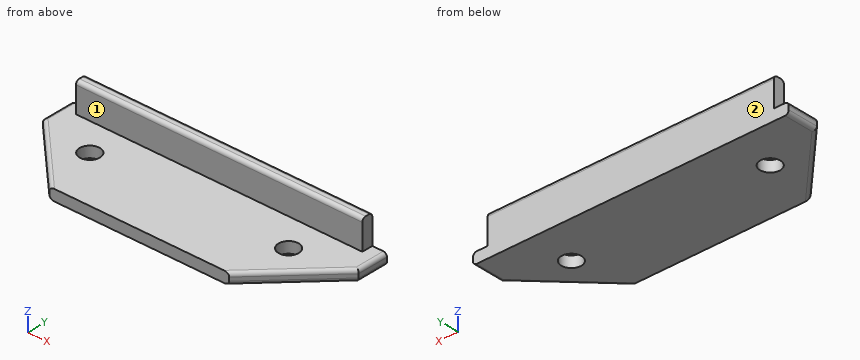
```python
from build123d import *

# Parameters (mm, degrees)
BOSS_EXTRUDE1_DEPTH       = 9.525
SKETCH2_W                 = 247.649999748
SKETCH2_H                 = 9.52499999
BOSS_EXTRUDE2_DEPTH       = 25.4
M16_CLEARANCE_HOLE1_D     = 17.462499982
M16_CLEARANCE_HOLE1_DEPTH = 34.925
FILLET1_R                 = 3.175


with BuildPart() as part:
    # Sketch1 → Boss-Extrude1 (new body)
    with BuildSketch(Plane.XY.offset(-7.9375)):
        Polygon((136.524999861, 15.874999984), (136.524999861, 42.862499956), (-136.524999861, 42.862499956), (-136.524999861, 15.874999984), (-77.787499921, -42.862499956), (77.787499921, -42.862499956), align=None)
    extrude(amount=-BOSS_EXTRUDE1_DEPTH)

    # Sketch2 → Boss-Extrude2 (add)
    with BuildSketch(Plane.XY.offset(-7.9375)):
        with Locations((0, 38.099999961)):
            Rectangle(SKETCH2_W, SKETCH2_H)
    extrude(amount=BOSS_EXTRUDE2_DEPTH)

    # M16 Clearance Hole1
    with Locations(Plane(origin=(0, 0, -17.4625), x_dir=(-1, 0, 0), z_dir=(0, 0, -1))):
        with Locations((-85.978999912, 4.762499995), (85.978999912, 4.762499995)):
            Hole(M16_CLEARANCE_HOLE1_D / 2, depth=M16_CLEARANCE_HOLE1_DEPTH)

    # Fillet1
    fillet1_edges = [part.edges().sort_by_distance(p)[0] for p in [
        (-136.524999861, 29.36874997, -17.4625),
        (-107.156249891, -13.493749986, -17.4625),
        (0, 33.337499966, 17.4625),
        (0, 42.862499956, 17.4625),
        (107.156249891, -13.493749986, -17.4625),
        (-107.156249891, -13.493749986, -7.9375),
        (-136.524999861, 29.36874997, -7.9375),
        (136.524999861, 29.36874997, -17.4625),
        (136.524999861, 29.36874997, -7.9375),
        (107.156249891, -13.493749986, -7.9375),
    ]]
    fillet(fillet1_edges, radius=FILLET1_R)


solid = part.part
```
Geometry check sheet. Reference: the model listing, model coordinates, mm. Face numbers are marked on the shaded views. A direction names the side the tool comes from. Round coordinates to 2 decimals unless told otherwise and drop trailing zeros. Order: outer loops, then holes, each group sorted by start corner. A loop starts at its lowest first (then second) coordinate and runs counter-clockwise, first axis right, second up. Notation, with made-up numbers: (54.25, 40.5) -> (107.25, 40.5) arc R19 ccw to (107.25, 66.5) -> close; hole circle Ø10 at (68, 77.25). An arc over 180 degrees is marked (long way). Return JSON: item names as keys, results as strings. Group by question number.
Q1. Material ranges on probe 1 along Z at (x, y) = (81, -6.5); probe 2 along Y at (x, z) = (-94, 12); probe 3 along Y at (x, z) = (-80, -12), recorded low to high. Write a range as from..to.
Q2. Tool access check on the marked faces 1 and 2. Record the directions out of +Z, -Z, +X, -X, +Y, -Y that give a thin tool (end or side, any length) a straight path to the whole face; none if there is none.
Q3. Section check C-C, the plane z = -1.5. Record the boundary of the cut face in (x, y) (1 decimal).
Q4. Gauge pin test, flat ends, axial feed: pin 1 (5 mm diameter, centred on y = 39, z = 5.5, fed in from -X) (3 decimals); pin 2 (2 mm diameter, centred on x = -98.5, z = -9, fed in from -Y); pin 3 (4 mm diameter, centred on x = -54, y = 29, fed in from +Z); pin 4 (15.5 mm diameter, centred on x = -85.98, y = 4.76, fed in from -Z). Record the tip position at first contact, or that the pin passes through.
Numbers:
{
 "1": {"probe 1": "-17.46..-7.94", "probe 2": "33.34..42.86", "probe 3": "-40.65..-1.6, 11.13..42.86"},
 "2": {"face 1": "+Z, +X, -X, -Y", "face 2": "+Z, -Z, +X, -X, +Y"},
 "3": {"outline": "(-123.8, 33.3) -> (123.8, 33.3) -> (123.8, 42.9) -> (-123.8, 42.9) -> close"},
 "4": {"pin 1": "x = -123.825", "pin 2": "y = -22.41", "pin 3": "z = -7.94", "pin 4": "through"}
}
